Input: part model. Units: mm. Frame: model coordinates. Face numbers are marked on the shaded views. A direction names the side the tool comes from. Round coordinates to 2 decimals unless told otherwise and drop trailing zeros. Order: outer loops, then holes, each group sorted by start corner. A loop starts at its lowest first (then second) coordinate and runs counter-clockwise, first axis right, second up. Notation, with made-up numbers: (-37, 26) -> (0, 26) arc R9 cw to (0, 41) -> close; hole circle Ø11 at (-16.5, 29). An arc over 180 degrees is marked (long way). Use a Markdown table: item, result.
Autodesk Inventor part; units mm, degrees
ref_plane "YZ Plane" through (0, 0, 0) normal (1, 0, 0) x (0, 1, 0)
ref_plane "XZ Plane" through (0, 0, 0) normal (0, 1, 0) x (-1, 0, 0)
ref_plane "XY Plane" through (0, 0, 0) normal (0, 0, 1) x (1, 0, 0)
sketch "Sketch1" plane through (0, 0, 0) normal (0, 1, 0) x (-1, 0, 0)
  line L0 (-119.8086, 12.5082) -> (-80.837, 16)
  line L1 (-80.837, 16) -> (0, 16)
  line L2 (-120, 0) -> (120, 0) construction
  line L3 (-120, -12.4911) -> (-80.837, -16)
  line L4 (-80.837, -16) -> (0, -16)
  line L5 (0, 16) -> (0, -16) construction
  line L6 (80.837, 16) -> (0, 16)
  line L7 (119.8086, 12.5082) -> (80.837, 16)
  line L8 (120, -12.4911) -> (80.837, -16)
  line L9 (80.837, -16) -> (0, -16)
  line L10 (-80.837, -12.486) -> (-114.3086, -9.487)
  line L11 (-80.837, 12.486) -> (-114.3086, 9.487)
  line L12 (-114.3086, 9.487) -> (-114.3086, -9.487)
  line L13 (-80.837, 12.486) -> (-80.837, -12.486)
  line L14 (-23, 12.5) -> (-43, 12.5)
  line L15 (-43, 12.5) -> (-43, -12.5)
  line L16 (-43, -12.5) -> (-23, -12.5)
  line L17 (-23, -12.5) -> (-23, 12.5)
  line L18 (80.837, -12.486) -> (114.3086, -9.487)
  line L19 (80.837, 12.486) -> (114.3086, 9.487)
  line L20 (114.3086, 9.487) -> (114.3086, -9.487)
  line L21 (80.837, 12.486) -> (80.837, -12.486)
  line L22 (23, 12.5) -> (43, 12.5)
  line L23 (43, 12.5) -> (43, -12.5)
  line L24 (43, -12.5) -> (23, -12.5)
  line L25 (23, -12.5) -> (23, 12.5)
  circle A0 centre (-17.5, -11) radius 1.5
  circle A1 centre (17.5, -11) radius 1.5
  circle A2 centre (-17.5, 11) radius 1.5
  circle A3 centre (17.5, 11) radius 1.5
  line L26 (-119.8086, 12.5082) -> (-158, 12.5082)
  line L27 (-158, 12.5082) -> (-158, -12.4911)
  line L28 (-120, -12.4911) -> (-158, -12.4911)
  circle A4 centre (-154.68, 0) radius 1.5
  line L29 (119.8086, 12.5082) -> (158, 12.5082)
  line L30 (158, 12.5082) -> (158, -12.4911)
  line L31 (120, -12.4911) -> (158, -12.4911)
  circle A5 centre (154.68, 0) radius 1.5
  point P0 (0, 0)
  point P1 (0, 0)
  point P2 (0, 0)
  point P3 (-114.3086, 0)
  point P4 (-33, 12.5)
  dimension "d0" = 25
  dimension "d2" = 80.837
  dimension "d6" = 3.5
  dimension "d9" = 3.5
  dimension "d10" = 3.5
  dimension "d11" = 20
  dimension "d13" = 3
  dimension "d14" = 5
  dimension "d15" = 5.5
  dimension "d17" = 38
  dimension "d18" = 39.163
  dimension "d19" = 5.5
  dimension "d23" = 3
  dimension "d24" = 3.32
  dimension "d30" = 32
  dimension "d33" = 23
  dimension "d34" = 3.5089
extrude "Extrusion1" add sketch "Sketch1" along normal mid plane 3
fillet "Fillet1" radius 3 2 edges at (-158, 0, 12.5082) (158, 0, 12.5082)
sketch "Sketch3" plane through (-80.837, 1.5, 16) normal (0, 0, 1) x (1, 0, 0)
  line L0 (0, 0) -> (161.674, 0)
  line L1 (161.674, -3) -> (0, -3)
  line L2 (57.837, -3) -> (57.837, 0)
  line L3 (103.837, -3) -> (103.837, 0)
  line L4 (57.837, -3) -> (57.837, 0)
  line L5 (57.837, -1.5) -> (103.837, -1.5)
  line L6 (238.837, -3) -> (238.837, 0)
  line L7 (200.6456, 0) -> (235.837, 0)
  line L8 (235.837, 0) -> (238.837, 0)
  line L9 (238.837, -3) -> (235.837, -3)
  line L10 (235.837, -3) -> (200.6456, -3)
  line L11 (200.6456, -3) -> (161.674, -3)
  line L12 (161.674, 0) -> (200.6456, 0)
  point P0 (80.837, -1.5)
extrude "Extrusion2" cut sketch "Sketch3" against normal through all contours L0 L12 L7 L8 L6 L9 L10 L11 L1 L3 | L5 L3 L1 L2
properties part number "nakladka" material "PCTG 20%"
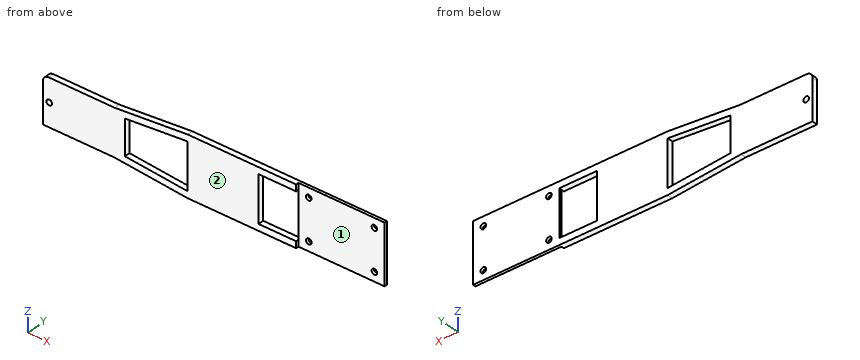
1) Cut plane B-B on z = -4.5. Return loops of the section in (x, y), and give its area (3 significant figures).
Results found:
| item | result |
|---|---|
| outline | (-158, -1.5) -> (-114.31, -1.5) -> (-114.31, 1.5) -> (-158, 1.5) -> close; (-80.84, -1.5) -> (-43, -1.5) -> (-43, 1.5) -> (-80.84, 1.5) -> close; (-23, 0) -> (23, 0) -> (23, 1.5) -> (-23, 1.5) -> close |
| area | 314 mm² |
2) Line query: L1, parallel to Z at x = 17.5, y = 0.3; L2, parallel to X at y = 0.1, z = -5; L3, parallel to Z at x = -42.5, y = -0.35. Output: solid intervals per line, ascending. Write a range as [from, to].
Results found:
| item | result |
|---|---|
| L1 | z = [-16, -12.5], [-9.5, 9.5], [12.5, 16] |
| L2 | x = [-158, -114.31], [-80.84, -43], [-23, 23] |
| L3 | z = [-16, -12.5], [12.5, 16] |
3) Set-up query: the marked faces 1 and 2. Return all of +Z, -Z, +X, -X, +Y, -Y with unobstructed straight access to the full face (end or side cutting, diameter ignored); none if empty.
Results found:
| item | result |
|---|---|
| face 1 | +Z, -Z, +X, -Y |
| face 2 | +Z, -Z, +X, -X, -Y |
4) Cut plane D-D on z = -11. Return loops of the section in (x, y).
Results found:
| item | result |
|---|---|
| outline | (-158, -1.5) -> (-97.42, -1.5) -> (-97.42, 1.5) -> (-158, 1.5) -> close; (-80.84, -1.5) -> (-43, -1.5) -> (-43, 1.5) -> (-80.84, 1.5) -> close; (-23, 0) -> (-19, 0) -> (-19, 1.5) -> (-23, 1.5) -> close; (-16, 0) -> (16, 0) -> (16, 1.5) -> (-16, 1.5) -> close; (19, 0) -> (23, 0) -> (23, 1.5) -> (19, 1.5) -> close |
5) Cut plane C-C on y = -0.9. Return loops of the section in (x, z), and give its area (3 significant figures).
Results found:
| item | result |
|---|---|
| outline | (-158, -12.49) -> (-120, -12.49) -> (-80.84, -16) -> (-23, -16) -> (-23, -12.5) -> (-43, -12.5) -> (-43, 12.5) -> (-23, 12.5) -> (-23, 16) -> (-80.84, 16) -> (-119.81, 12.51) -> (-155, 12.51) arc R3 ccw to (-158, 9.51) -> close; hole circle Ø3 at (-154.68, 0); hole (-114.31, -9.49) -> (-80.84, -12.49) -> (-80.84, 12.49) -> (-114.31, 9.49) -> close |
| area | 2,670 mm² |
6) Cut plane A-A on x = -30.5. Return loops of the section in (y, z), and give its area (3 significant figures).
Results found:
| item | result |
|---|---|
| outline | (-1.5, -16) -> (1.5, -16) -> (1.5, -12.5) -> (-1.5, -12.5) -> close; (-1.5, 12.5) -> (1.5, 12.5) -> (1.5, 16) -> (-1.5, 16) -> close |
| area | 21.0 mm² |
7) Pin query (flat end, axial travel): pin 1 Ø2.5 at (x, z) = (-17.5, 11) entering from -Y; pin 2 Ø0.8 at (y, z) = (-1, -13.5) entering from +X; pin 3 Ø16 at (x, z) = (4.5, -6) entering from -Y. Return the tip coordinate at first contact, or that it passes through.
Results found:
| item | result |
|---|---|
| pin 1 | passes through |
| pin 2 | stops at x = -23 |
| pin 3 | stops at y = 0 |
